Autodesk Inventor part; units mm, degrees
ref_plane "YZ Plane" through (0, 0, 0) normal (1, 0, 0) x (0, 1, 0)
ref_plane "XZ Plane" through (0, 0, 0) normal (0, 1, 0) x (-1, 0, 0)
ref_plane "XY Plane" through (0, 0, 0) normal (0, 0, 1) x (1, 0, 0)
sketch "Sketch1" plane through (0, 0, 0) normal (0, 1, 0) x (-1, 0, 0)
  line L0 (-20, 11) -> (20, 11)
  line L1 (20, 11) -> (20, -11)
  line L2 (20, -11) -> (-20, -11)
  line L3 (-20, -11) -> (-20, 11)
  line L4 (-20, 11) -> (20, -11) construction
  line L5 (20, 11) -> (-20, -11) construction
  point P0 (0, 0)
  dimension "d0" = 40
  dimension "d1" = 22
extrude "Extrusion1" add sketch "Sketch1" along normal blind 20
fillet "Fillet1" radius 4 8 edges at (0, 20, 11) (20, 20, 0) (20, 10, 11) (20, 10, -11) (0, 20, -11) (-20, 10, -11) (-20, 20, 0) (-20, 10, 11)
sketch "Sketch2" plane through (20, 0, 7) normal (1, 0, 0) x (0, 0, -1)
  line L0 (14, 0) -> (0, 0) construction
  line L1 (14, 16) -> (18, 16) construction
  line L2 (0, 0) -> (14, 16) construction
  line L3 (14, 16) -> (0, 16) construction
  line L4 (0, 16) -> (14, 0) construction
  line L5 (9, 8.75) -> (5, 8.75)
  line L6 (5, 8.75) -> (5, 7.25)
  line L7 (5, 7.25) -> (9, 7.25)
  line L8 (9, 7.25) -> (9, 8.75)
  line L9 (9, 8.75) -> (5, 7.25) construction
  line L10 (5, 8.75) -> (9, 7.25) construction
  point P0 (7, 0)
  point P1 (7, 8)
  dimension "d5" = 4
  dimension "d6" = 1.5
extrude "Extrusion2" add sketch "Sketch2" along normal blind 3
sketch "Sketch3" plane through (0, 0, 0) normal (0, -1, 0) x (1, 0, 0)
  arc A0 (20, 7) -> (16, 11) centre (16, 7) ccw
  arc A1 (-20, -7) -> (-16, -11) centre (-16, -7) ccw
  line L0 (16, 7) -> (-16, -7) construction
  line L1 (-16, 7) -> (-16, 11)
  line L2 (-16, -7) -> (-16, 7) construction
  line L3 (20, -7) -> (16, -7)
  line L4 (-16, 7) -> (16, -7) construction
  line L5 (16, -7) -> (16, 7) construction
  line L6 (16, 7) -> (11, 7) construction
  line L7 (16, 7) -> (-16, 7) construction
  line L8 (11, 7) -> (11, -7) construction
  circle A2 centre (11, 0) radius 2.5
  point P0 (0, 0)
  dimension "d9" = 5
  dimension "d10" = 5
extrude "Extrusion3" add sketch "Sketch3" along normal blind 2
sketch "Sketch4" plane through (11, -2, 0) normal (0, -1, 0) x (1, 0, 0)
  line L0 (-1.3, -4.4849) -> (1.3, -4.4849)
  line L1 (1.3, -2.1354) -> (1.3, 2.1354)
  line L2 (-1.3, 2.1354) -> (-1.3, -2.1354)
  line L3 (-1.3, -4.4849) -> (1.3, 4.4849) construction
  line L4 (1.3, -4.4849) -> (-1.3, 4.4849) construction
  circle A0 centre (0, 0) radius 2.5
  arc A1 (1.3, 2.1354) -> (-1.3, 2.1354) centre (0, 0) ccw
  arc A2 (-1.3, -2.1354) -> (1.3, -2.1354) centre (0, 0) ccw
  point P0 (-11, 0)
  dimension "d13" = 2.6
extrude "Extrusion4" add sketch "Sketch4" along normal blind 2 contours A0 L2 L1
sketch "Sketch5" plane through (-20, 0, -7) normal (-1, 0, 0) x (0, 0, 1)
  line L0 (5, 8.75) -> (9, 8.75)
  circle A0 centre (7, 8.75) radius 7.0401
  point P0 (7, 0)
extrude "Extrusion5" add sketch "Sketch5" along normal blind 11
ref_plane "Work Plane1" through (-16, 0, 0) normal (0, 0, 1) x (1, 0, 0)
properties part number "Lifting Motor"
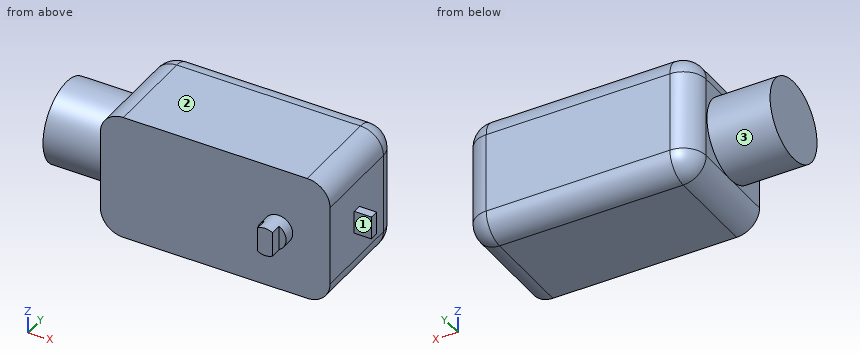
Could you check a few things on this model? Use its own coordinates, in mm. Face numbers are marked on the shaded views. A direction names the side the tool comes from. Round coordinates to 2 decimals unless told otherwise and drop trailing zeros. Order: outer loops, then holes, each group sorted by start corner. A loop starts at its lowest first (then second) coordinate and runs counter-clockwise, first axis right, second up. Notation, with made-up numbers: M 27,6.5 L 80,6.5 A30 cw 80,34.5 Z; hole C -7,29 d8. An arc over 180 degrees is marked long. One line per question, with ' | ' between items. Start each with the question number.
(1) Suppose I cut it at A-A on z = 0. List the corners of the cut face in (x, y) for me.
(2) Please list where these lines run through material, in increasing order: line 1 along Y through (x, z) = (9.5, 0.25); line 2 along Y through (x, z) = (-9, -6.5); line 3 along X through (y, z) = (16, -4.75).
(3) For the marked faces 1, 2 and 3, which set-ups out of +Z, -Z, +X, -X, +Y, -Y let a thin tool reach every point of the face, with its end or its side?
(4) For P1, Ø6, axis at y = 4, z = 3.5, coming from the +X side; P2, Ø5, axis at x = 7.5, z = 8, coming from the -Y side; P3, Ø1.5, axis at x = -25.5, y = 7.5, coming from the -Z side, each with a flat end and sliding along its axis, tell me the tip position at first contact or that it passes through.
(5) Suppose I cut it at D-D on y = 12.75. List the corners of the cut face in (x, z) for me.
(6) Suppose I cut it at B-B on x = 7.5. List the corners of the cut face in (y, z) for me, then the cut area to 3 significant figures.
(7) Suppose I cut it at C-C on y = 5. List the corners of the cut face in (x, z) for me, then the cut area to 3 significant figures.
Geometry results:
1) outline: M -31,1.71 L -20,1.71 L -20,0 L 8.5,0 L 8.5,-2 L 9.7,-2 L 9.7,-4 L 12.3,-4 L 12.3,-2 L 13.5,-2 L 13.5,0 L 20,0 L 20,7.25 L 23,7.25 L 23,8.75 L 20,8.75 L 20,16 A4 ccw 16,20 L -16,20 A4 ccw -20,16 L -20,15.79 L -31,15.79 Z
2) line 1: -2 to 20 | line 2: 0 to 20 | line 3: -20 to 20
3) face 1: +Z, -Z, +X, -Y | face 2: +Z, +X, -X, +Y, -Y | face 3: -X
4) P1: x = 20 | P2: y = 0 | P3: z = -7.02
5) outline: M -31,-5.79 L -20,-5.79 L -20,-7 A4 ccw -16,-11 L 16,-11 A4 ccw 20,-7 L 20,7 A4 ccw 16,11 L -16,11 A4 ccw -20,7 L -20,5.79 L -31,5.79 Z
6) outline: M 0,-11 L 16,-11 A4 ccw 20,-7 L 20,7 A4 ccw 16,11 L 0,11 Z | area: 433 mm²
7) outline: M -31,-5.96 L -20,-5.96 L -20,-7 A4 ccw -16,-11 L 16,-11 A4 ccw 20,-7 L 20,7 A4 ccw 16,11 L -16,11 A4 ccw -20,7 L -20,5.96 L -31,5.96 Z | area: 997 mm²
